For this review, take the finished solid that the model builds, in its own axes (mm). Face numbers are marked on the shaded views. A direction names the side the tool comes from. Coordinates: 2 decimals unless noted, no trailing zeros. Loops run counter-clockwise (first coordinate to the right, second up) from the corner with the lowest first, then second, coordinate; pieces in that order, holes last. Notation, with made-up numbers: M 12.25,87.5 L 53.25,87.5 A31 ccw 53.25,124.5 Z; hole C 44,-1.5 d7. An arc over 180 degrees is marked long. Write item = value, one per line.
from build123d import *

# Parameters (mm, degrees)
F0_R        = 1.3671138527
F0_R_2      = 1.4471777078
F0_W        = 46.99
F0_H        = 38.1
F0_R_3      = 1.4536013708
F0_R_4      = 1.3946138209
F1_DEPTH    = 15.24
F2_T        = 2.54
F2_T3_DEPTH = 20.32


# Not quite as in the source:
# - a shell that OpenCascade refuses in one call is made with other operations: the cavity is built on its own and cut out


with BuildPart() as f1:
    # F0 (on Top) → F1 (new body)
    with BuildSketch(Plane.XY):
        Polygon((0, 46.99), (0, 44.45), (16.51, 44.45), (63.5, 44.45), (76.2, 44.45), (76.2, 46.99), (76.2, 50.8), (72.39, 50.8), (3.81, 50.8), (0, 50.8), align=None)
        with Locations((3.81, 46.99)):
            Circle(F0_R, mode=Mode.SUBTRACT)
        with Locations((72.39, 46.99)):
            Circle(F0_R_2, mode=Mode.SUBTRACT)
        with Locations((40.005, 25.4)):
            Rectangle(F0_W, F0_H)
        Polygon((0, 3.175), (0, 0), (3.81, 0), (72.39, 0), (76.2, 0), (76.2, 3.81), (76.2, 6.35), (63.5, 6.35), (16.51, 6.35), (0, 6.35), (0, 3.81), align=None)
        with Locations((3.81, 3.81)):
            Circle(F0_R_3, mode=Mode.SUBTRACT)
        with Locations((72.39, 3.81)):
            Circle(F0_R_4, mode=Mode.SUBTRACT)
    extrude(amount=F1_DEPTH)

    # F2: shell of thickness 2.54, made by hand


with BuildPart() as f2_core1:
    # F2_t2: copy of F1
    add(f1.part)

    # the walls: a layer under each face that stays
    f2_faces = [f2_core1.faces().sort_by_distance(p)[0] for p in [
        (8.255, 44.45, 7.62),
        (16.51, 25.4, 7.62),
        (8.255, 6.35, 7.62),
        (0, 3.175, 7.62),
        (38.1, 0, 7.62),
        (76.2, 3.175, 7.62),
        (69.85, 6.35, 7.62),
        (63.5, 25.4, 7.62),
        (69.85, 44.45, 7.62),
        (76.2, 47.625, 7.62),
        (38.1, 50.8, 7.62),
        (0, 47.625, 7.62),
        (2.4428861473, 46.99, 7.62),
        (70.9428222922, 46.99, 7.62),
        (70.9953861791, 3.81, 7.62),
        (2.3563986292, 3.81, 7.62),
        (38.1, 25.4, 15.24),
    ]]
    thicken(f2_faces, amount=-F2_T, mode=Mode.SUBTRACT)

    # F2_s4 → F2_t3 (cut)
    with BuildSketch(Plane.XY.offset(-2.54)):
        Polygon((16.4846, 44.4246), (16.51, 46.99), (19.05, 46.99), (19.05, 44.45), align=None)
        Polygon((16.4846, 6.3754), (19.05, 6.35), (19.05, 3.81), (16.51, 3.81), align=None)
        Polygon((63.5254, 6.3754), (63.5, 3.81), (60.96, 3.81), (60.96, 6.35), align=None)
        Polygon((63.5254, 44.4246), (60.96, 44.45), (60.96, 46.99), (63.5, 46.99), align=None)
    extrude(amount=F2_T3_DEPTH, mode=Mode.SUBTRACT)


with BuildPart() as f1_1:
    add(f1.part)

    # what is left inside the walls is the cavity
    f2_cavity = [f2_core1.part.solids().sort_by_distance(p)[0] for p in [
        (38.085466, 17.78, 0.0254),
    ]]
    add(f2_cavity, mode=Mode.SUBTRACT)


solid = f1_1.part
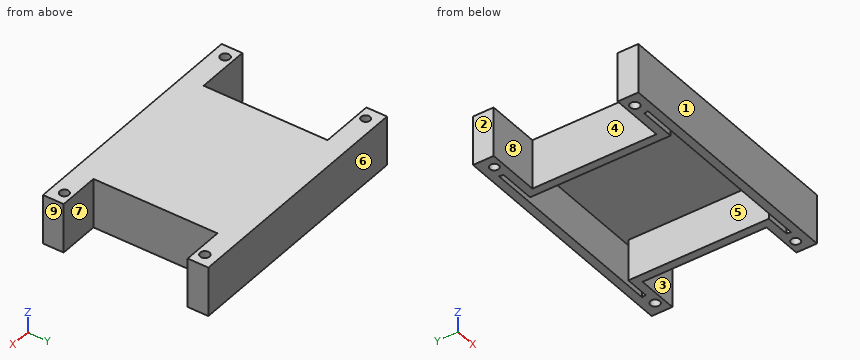
Q1. For pin 1 Ø3 at (x, y) = (47.5, 45) entering from -Z; pin 2 Ø1.5 at (y, z) = (21, 3) entering from -X; pin 3 Ø2 at (y, z) = (39, 10) entering from +X, all flat-tipped, find the tip position at first contact; note any pin that passes through.
Solved:
pin_1 = 12.7
pin_2 = 16.51
pin_3 = 63.5
Q2. Add section B-B (x = 15.5). Write out the cut boundary in (y, z), and give its area (3 significant figures).
Solved:
outline = M 0,0 L 2.54,0 L 2.54,12.7 L 3.81,12.7 L 3.81,0 L 6.35,0 L 6.35,15.24 L 0,15.24 Z; M 44.45,0 L 46.99,0 L 46.99,12.7 L 48.26,12.7 L 48.26,0 L 50.8,0 L 50.8,15.24 L 44.45,15.24 Z
area = 161 mm²
Q3. Add section D-D (z = 9.25). Write out the cut boundary in (x, y).
Solved:
outline = M 0,0 L 76.2,0 L 76.2,6.35 L 63.5,6.35 L 63.5,44.45 L 76.2,44.45 L 76.2,50.8 L 0,50.8 L 0,44.45 L 16.51,44.45 L 16.51,6.35 L 0,6.35 Z; hole C 3.81,3.81 d2.91; hole C 3.81,46.99 d2.73; hole M 7.5,48.26 A3.91 cw 7.72,46.99 L 19.05,46.99 L 19.05,3.81 L 7.8,3.81 A3.99 cw 7.6,2.54 L 68.67,2.54 A3.93 cw 68.46,3.81 L 60.96,3.81 L 60.96,46.99 L 68.4,46.99 A3.99 cw 68.61,48.26 Z; hole C 72.39,46.99 d2.89; hole C 72.39,3.81 d2.79
Q4. Draft analysis for pull direction Y (two halves, no side actions). For the marked faces 1, 2, 3 and 4, state which applies: +Y half, -Y half, draft (parallel to the pull), parting line (faces both ways), or undercut.
Solved:
face_1 = -Y half
face_2 = draft
face_3 = undercut
face_4 = undercut
Q5. Machinability: for the marked faces 5, 6, 7, 8 and 9, which of the approach directions +Z, -Z, +X, -X, +Y, -Y give a long, thin tool a straight path to every point of the face, cutting with its end or side? Answer none if there is none.
Solved:
face_5 = -Z
face_6 = +Z, -Z, +X, -X, +Y
face_7 = +Z, -Z, +X
face_8 = +Z, -Z, -X
face_9 = +Z, -Z, +X, +Y, -Y
Q6. For line 1 along Y through (x, z) = (3.81, 8.25); line 2 along Y through (x, z) = (62.5, 6.25); line 3 along Y through (x, z) = (58.5, 9), list the stretches that pass through material, from the lowest coordinate up.
Solved:
line_1 = 0 to 2.36, 5.26 to 6.35, 44.45 to 45.62, 48.36 to 50.8
line_2 = 0 to 2.54, 3.81 to 46.99, 48.26 to 50.8
line_3 = 0 to 2.54, 48.26 to 50.8
Q7. Add section A-A (x = 72.39). Write out the cut boundary in (y, z), and give its area (3 significant figures).
Solved:
outline = M 0,0 L 2.42,0 L 2.42,15.24 L 0,15.24 Z; M 5.2,0 L 6.35,0 L 6.35,15.24 L 5.2,15.24 Z; M 44.45,0 L 45.54,0 L 45.54,15.24 L 44.45,15.24 Z; M 48.44,0 L 50.8,0 L 50.8,15.24 L 48.44,15.24 Z
area = 107 mm²
Q8. Add section C-C (y = 34.5). Write out the cut boundary in (x, z), and give its area (3 significant figures).
Solved:
outline = M 16.51,0 L 19.05,0 L 19.05,12.7 L 60.96,12.7 L 60.96,0 L 63.5,0 L 63.5,15.24 L 16.51,15.24 Z
area = 184 mm²
